from build123d import *

# Parameters (mm, degrees)
SKETCH_1_W          = 80
SKETCH_1_H          = 80
EXTRUDE_1_DEPTH     = 10
FILLET_1_R          = 10
SKETCH_2_W          = 10
SKETCH_2_H          = 10
CUT_EXTRUDE_1_DEPTH = 8
CUT_EXTRUDE_2_DEPTH = 58.445626465
SKETCH_4_R          = 5
EXTRUDE_2_DEPTH     = 60


with BuildPart() as part:
    # ｽｹｯﾁ1 → ﾎﾞｽ - 押し出し1 (new body)
    with BuildSketch(Plane(origin=(0, 0, 0), x_dir=(1, 0, 0), z_dir=(0, 1, 0))):
        Rectangle(SKETCH_1_W, SKETCH_1_H)
    extrude(amount=EXTRUDE_1_DEPTH)

    # ﾌｨﾚｯﾄ1
    fillet_1_edges = [part.edges().sort_by_distance(p)[0] for p in [
        (40, 5, 40),
        (-40, 5, 40),
        (-40, 5, -40),
        (40, 5, -40),
    ]]
    fillet(fillet_1_edges, radius=FILLET_1_R)

    # ｽｹｯﾁ2 → ｶｯﾄ - 押し出し1 (cut)
    with BuildSketch(Plane(origin=(0, 0, 0), x_dir=(1, 0, 0), z_dir=(0, 1, 0))):
        with Locations((-27, 0)):
            Rectangle(SKETCH_2_W, SKETCH_2_H)
        with Locations((27, 0)):
            Rectangle(SKETCH_2_W, SKETCH_2_H)
    extrude(amount=CUT_EXTRUDE_1_DEPTH, mode=Mode.SUBTRACT)

    # ｽｹｯﾁ3 → ｶｯﾄ - 押し出し2 (cut, through all)
    with BuildSketch(Plane(origin=(0, 10, 0), x_dir=(1, 0, 0), z_dir=(0, 1, 0))):
        with BuildLine():
            Line((-4, -25), (4, -25))
            ThreePointArc((4, -25), (11.071067812, -22.071067812), (14, -15))
            Line((14, -15), (14, 15))
            ThreePointArc((14, 15), (11.071067812, 22.071067812), (4, 25))
            Line((4, 25), (-4, 25))
            ThreePointArc((-4, 25), (-11.071067812, 22.071067812), (-14, 15))
            Line((-14, 15), (-14, -15))
            ThreePointArc((-14, -15), (-11.071067812, -22.071067812), (-4, -25))
        make_face()
    extrude(amount=-CUT_EXTRUDE_2_DEPTH, mode=Mode.SUBTRACT)

    # ｽｹｯﾁ4 → ﾎﾞｽ - 押し出し2 (add)
    with BuildSketch(Plane(origin=(0, 10, 0), x_dir=(1, 0, 0), z_dir=(0, 1, 0))):
        with Locations(Location((-30, 30, 0), (0, 0, 90))):
            Circle(SKETCH_4_R)
        with Locations(Location((30, 30, 0), (0, 0, 90))):
            Circle(SKETCH_4_R)
        with Locations(Location((-30, -30, 0), (0, 0, 90))):
            Circle(SKETCH_4_R)
        with Locations(Location((30, -30, 0), (0, 0, 90))):
            Circle(SKETCH_4_R)
    extrude(amount=EXTRUDE_2_DEPTH)


solid = part.part
The listing builds one solid part. Answer for the finished solid, in the listing's coordinates (mm). A direction names the side the tool comes from. Give positions to 0.01 mm unless a question says otherwise; leave off trailing zeros. Write each loop counter-clockwise with the first axis right and the second up, starting at its lowest first coordinate (ties: lowest second). Pieces come first, ordered by that corner, then holes. Notation, with made-up numbers: (48, -34.5) -> (107, -34.5) arc R25 cw to (107, -17.5) -> close; hole circle Ø1 at (80.5, 82). An arc over 180 degrees is marked (long way). Use a Markdown table: item, result.
(1) Section D-D, the plane y = 42.5 is taken. Determine the outline of the cut face in (x, z).
Return value:
| item | result |
|---|---|
| outline | circle Ø10 at (-30, -30); circle Ø10 at (-30, 30); circle Ø10 at (30, -30); circle Ø10 at (30, 30) |
(2) Section B-B, the plane x = 0.5 is taken. Determine the outline of the cut face in (y, z).
Return value:
| item | result |
|---|---|
| outline | (0, -40) -> (10, -40) -> (10, -25) -> (0, -25) -> close; (0, 25) -> (10, 25) -> (10, 40) -> (0, 40) -> close |
(3) Find the intervals of material crossed by probe 1 along Y at (x, z) = (21, -25.5); probe 2 along X at (y, z) = (43, -31); probe 3 along Z at (x, y) = (6, 8), in increasing order. Write a range as from..to.
Return value:
| item | result |
|---|---|
| probe 1 | 0..10 |
| probe 2 | -34.9..-25.1, 25.1..34.9 |
| probe 3 | -40..-24.8, 24.8..40 |
(4) Section A-A, the plane z = 12 is taken. Determine the outline of the cut face in (x, y), then the cut area to 3 significant figures.
Return value:
| item | result |
|---|---|
| outline | (-40, 0) -> (-14, 0) -> (-14, 10) -> (-40, 10) -> close; (14, 0) -> (40, 0) -> (40, 10) -> (14, 10) -> close |
| area | 520 mm2 |
(5) Section C-C, the plane z = -3 is taken. Determine the outline of the cut face in (x, y), then the cut area to 3 significant figures.
Return value:
| item | result |
|---|---|
| outline | (-40, 0) -> (-32, 0) -> (-32, 8) -> (-22, 8) -> (-22, 0) -> (-14, 0) -> (-14, 10) -> (-40, 10) -> close; (14, 0) -> (22, 0) -> (22, 8) -> (32, 8) -> (32, 0) -> (40, 0) -> (40, 10) -> (14, 10) -> close |
| area | 360 mm2 |
(6) For faces 4 (the flat face through (0, 5, 40)), 5 (the flat face through (0, 5, 25)), 6 (the flat face through (27, 8, 0)), determine the directions among +Z, -Z, +X, -X, +Y, -Y from which every point of the face is accessible in a straight line to the end or side of a thin tool.
Return value:
| item | result |
|---|---|
| face 4 | +Z, +X, -X, +Y, -Y |
| face 5 | +Y, -Y |
| face 6 | -Y |
(7) Determine the mould class of faces 1 (the flat face through (-40, 5, 0)), 2 (the flat face through (17, 10, -1)), 3 (the cylindrical face through (36.99, 5.07, 37.15)) for opening direction X: released by +X, released by -X, zero draft, split by the parting line, or undercut.
Return value:
| item | result |
|---|---|
| face 1 | released by -X |
| face 2 | undercut |
| face 3 | released by +X |
(8) Flat-ended cylindrical pins translate along their axes: P1, Ø24, axis at x = 4.5, z = -8.5, coming from the +Y side; P2, Ø5, axis at x = -29, z = -1, coming from the -Y side. Find the tip coordinate at first contact, or state that the pin passes through.
Return value:
| item | result |
|---|---|
| P1 | y = 10 |
| P2 | y = 8 |
